```python
from build123d import *

# Parameters (mm, degrees)
SKETCH1_W           = 7.5
SKETCH1_H           = 5
SKETCH1_W_2         = 20
SKETCH1_W_3         = 15
BOSS_EXTRUDE1_DEPTH = 5


with BuildPart() as part:
    # Sketch1 → Boss-Extrude1 (new body)
    with BuildSketch(Plane.XY):
        Polygon((480, 177.5), (485, 177.5), (485, 187.5), (480, 187.5), (480, 190), (472.5, 190), (472.5, 195), (480, 195), (480, 200), (447.5, 200), (447.5, 195), (377.5, 195), (377.5, 200), (337.5, 200), (337.5, 195), (217.5, 195), (217.5, 200), (177.5, 200), (177.5, 195), (107.5, 195), (107.5, 200), (75, 200), (75, 195), (75, 187.5), (70, 187.5), (70, 177.5), (75, 177.5), (75, 170), (480, 170), align=None)
        with Locations((453.75, 192.5)):
            Rectangle(SKETCH1_W, SKETCH1_H, mode=Mode.SUBTRACT)
        with Locations((95, 182.5)):
            Rectangle(SKETCH1_W_2, SKETCH1_H, mode=Mode.SUBTRACT)
        with Locations((304.5, 182.5)):
            Rectangle(SKETCH1_W_3, SKETCH1_H, mode=Mode.SUBTRACT)
        with Locations((275.5, 182.5)):
            Rectangle(SKETCH1_W_3, SKETCH1_H, mode=Mode.SUBTRACT)
    extrude(amount=BOSS_EXTRUDE1_DEPTH)


solid = part.part
```
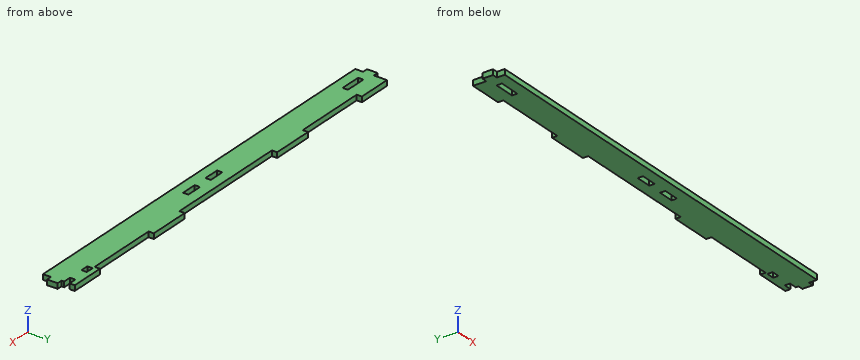
Verification items for the finished model (mm, model axes). Coordinates: 2 decimals unless noted, no trailing zeros. Loops run counter-clockwise (first coordinate to the right, second up) from the corner with the lowest first, then second, coordinate; pieces in that order, holes last. Notation, with made-up numbers: (-20, 47.5) -> (13, 47.5) arc R19 ccw to (13, 76.5) -> close; hole circle Ø7 at (75, -25.75). An arc over 180 degrees is marked (long way). Answer in a Markdown table with one row per item. Add a question column.
1. Section check C-C, the plane y = 173.75. Enter the section's corners in (x, z), then the cut area to 4 significant figures.
2. Section check A-A, the plane x = 159.5. Enter the section's corners in (y, z).
3. Section check B-B, the plane z = 3.5. Give the number of separate pieces and of enclosed holes in the cut face, then the cut area to 3 significant figures.
4. Depth check by flat-ended pin: P1, Ø2.5, axis at y = 197, z = 3, coming from the +X side; P2, Ø1.5, axis at x = 71.5, z = 3, coming from the +Y side. Enter the tip coordinate at first touch or a pass-through.
5. Material ranges on probe 1 along X at (y, z) = (180.25, 2); probe 2 along X at (y, z) = (195.75, 4.7); probe 3 along Y at (x, z) = (88, 3.5), recorded low to high. Write a range as [from, to].
Derived:
| question | item | result |
|---|---|---|
| 1 | outline | (75, 0) -> (480, 0) -> (480, 5) -> (75, 5) -> close |
| 1 | area | 2,025 mm² |
| 2 | outline | (170, 0) -> (195, 0) -> (195, 5) -> (170, 5) -> close |
| 3 | separate pieces | 1 |
| 3 | enclosed holes | 4 |
| 3 | area | 10,600 mm² |
| 4 | P1 | stops at x = 480 |
| 4 | P2 | stops at y = 187.5 |
| 5 | probe 1 | x = [70, 85], [105, 268], [283, 297], [312, 485] |
| 5 | probe 2 | x = [75, 107.5], [177.5, 217.5], [337.5, 377.5], [447.5, 480] |
| 5 | probe 3 | y = [170, 180], [185, 200] |
